For this review, take the finished solid that the model builds, in its own axes (mm). A direction names the side the tool comes from. Coordinates: 2 decimals unless noted, no trailing zeros. Order: outer loops, then holes, each group sorted by start corner. A loop starts at its lowest first (then second) coordinate and runs counter-clockwise, first axis right, second up. Notation, with made-up numbers: (2.25, 65) -> (34.25, 65) arc R34 ccw to (34.25, 101) -> close; hole circle Ø9 at (6.25, 47). An arc over 180 degrees is marked (long way). Answer as a JSON object with one key per item and string values. Group by question number.
1) Add section A-A, the plane z = 9.5. Write out the cut boundary in (x, y), then the cut area to 3 significant figures.
2) Wall thickness on L1, parallel to Y at x = 356.5, z = 1.95; L2, parallel to X at y = 387.5, z = 1.8; L3, parallel to X at y = 309, z = 9.5: over which ranges is each line inside the solid? List them lowest first.
3) Machinability: for faces 1 (the flat face through (173, 317, 3)), 2 (the flat face through (340, 388, 9)), 3 (the flat face through (179, 239.5, 6)), which of the approach directions +Z, -Z, +X, -X, +Y, -Y give a long, thin tool a straight path to every point of the face, cutting with its end or side? Answer none if there is none.
4) For pin 1 (3 mm diameter, centred on x = -5, y = 243.5, fed in from -Z); pin 2 (5 mm diameter, centred on x = 31.5, y = 335.5, fed in from +Z); pin 3 (10.5 mm diameter, centred on x = 328.5, y = 387, fed in from +Z), all flat-tipped, find the tip position at first contact; note any pin that passes through.
5) Add section C-C, the plane x = 237.5. Write out the cut boundary in (y, z), then the cut area to 3 significant figures.
6) Draft analysis for pull direction Y (two halves, no side actions). For faces 4 (the flat face through (173, 392.5, 6)), 5 (the flat face through (0, 317, 8)), 6 (the flat face through (-9.5, 315, 6)), state which applies: +Y half, -Y half, draft (parallel to the pull), parting line (faces both ways), or undercut.
7) Add section B-B, the plane y = 360. Write out the cut boundary in (x, z), then the cut area to 3 significant figures.
Autodesk Fusion 360 part; units mm, degrees
sketch "Sketch1" plane through (0, 0, 0) normal (0, 0, 1) x (1, 0, 0)
  line L0 (0, 250) -> (351, 250)
  line L1 (351, 250) -> (351, 383)
  line L2 (351, 383) -> (0, 383)
  line L3 (0, 383) -> (0, 250)
  line L4 (-9.5, 392.5) -> (361.5, 392.5)
  line L5 (361.5, 392.5) -> (361.5, 239.5)
  line L6 (361.5, 239.5) -> (-9.5, 239.5)
  line L7 (-9.5, 239.5) -> (-9.5, 392.5)
  circle A0 centre (-4.5, 244.5) radius 1.7
  circle A1 centre (356.5, 244.5) radius 1.7
  circle A2 centre (-4.5, 387.5) radius 1.7
  circle A3 centre (356.5, 387.5) radius 1.7
  circle A4 centre (-4.5, 387.5) radius 3
  circle A5 centre (356.5, 244.5) radius 3
  circle A6 centre (-4.5, 244.5) radius 3
  circle A7 centre (356.5, 387.5) radius 3
  dimension "d1" = 351
  dimension "d2" = 133
  dimension "d3" = 371
  dimension "d4" = 153
  dimension "d5" = 9.5
  dimension "d10" = 9.5
  dimension "d11" = 3.4
  dimension "d12" = 5
  dimension "d13" = 5
  dimension "d14" = 3.4
  dimension "d15" = 5
  dimension "d16" = 5
  dimension "d17" = 3.4
  dimension "d18" = 5
  dimension "d19" = 5
  dimension "d21" = 5
  dimension "d22" = 5
  dimension "d23" = 6
  dimension "d24" = 6
  dimension "d25" = 6
  dimension "d26" = 6
extrude "Extrude1" add sketch "Sketch1" along normal blind 10 from surface at 3.1 contours A4 | A5 | A6 | A7 makes body 1 at (-1.5928, 245.2403, 9.7667) makes body 2 at (357.3125, 247.3879, 9.7667) makes body 3 at (-7.0599, 389.0643, 9.7667) makes body 4 at (355.1314, 384.8304, 6.4333)
extrude "Extrude2" add sketch "Sketch1" along normal blind 13 contours L4 L5 L6 L7 bodies 1 2 3 4
extrude "Extrude3" add sketch "Sketch1" along normal blind 3 contours L0 L1 L2 L3 bodies 1
sketch "Sketch2" plane through (0, 0, 13) normal (0, 0, 1) x (-1, 0, 0)
  line L0 (0, -250) -> (0, -383)
  line L1 (0, -383) -> (-351, -383)
  line L2 (-351, -383) -> (-351, -250)
  line L3 (-351, -250) -> (0, -250)
  circle A0 centre (-356.5, -244.5) radius 3
  circle A1 centre (4.5, -244.5) radius 3
  circle A2 centre (4.5, -387.5) radius 3
  circle A3 centre (-356.5, -387.5) radius 3
  line L4 (9.5, -239.5) -> (-361.5, -239.5)
  line L5 (-361.5, -239.5) -> (-361.5, -392.5)
  line L6 (-361.5, -392.5) -> (9.5, -392.5)
  line L7 (9.5, -392.5) -> (9.5, -239.5)
sketch "Sketch3" plane through (0, 0, 13) normal (0, 0, 1) x (-1, 0, 0)
  line L0 (2440, -1230) -> (2470, -1230)
  line L1 (2470, -1230) -> (2470, -1260)
  line L2 (2470, -1260) -> (2440, -1260)
  line L3 (2440, -1260) -> (2440, -1230)
sketch "Sketch4" plane through (0, 0, 0) normal (1, 0, 0) x (0, 1, 0)
sketch "Sketch5" plane through (0, 0, 0) normal (0, 0, 1) x (1, 0, 0)
extrude "Extrude4" cut sketch "Sketch3" against normal blind 7.5 bodies 1
sketch "Sketch6" plane through (0, 0, 13) normal (0, 0, 1) x (-1, 0, 0)
  line L0 (-320, -400) -> (-340, -400)
  line L1 (-340, -400) -> (-340, -380)
  line L2 (-340, -380) -> (-320, -380)
  line L3 (-320, -380) -> (-320, -400)
extrude "Extrude5" cut sketch "Sketch6" against normal blind 7.5 bodies 1
Output values:
{
 "1": {"outline": "(-9.5, 239.5) -> (361.5, 239.5) -> (361.5, 392.5) -> (340, 392.5) -> (340, 383) -> (351, 383) -> (351, 250) -> (0, 250) -> (0, 383) -> (320, 383) -> (320, 392.5) -> (-9.5, 392.5) -> close; hole circle Ø3.4 at (-4.5, 244.5); hole circle Ø3.4 at (-4.5, 387.5); hole circle Ø3.4 at (356.5, 244.5); hole circle Ø3.4 at (356.5, 387.5)", "area": "9,850 mm²"},
 "2": {"L1": "y = 239.5 to 241.5, 247.5 to 384.5, 390.5 to 392.5", "L2": "x = -9.5 to -7.5, -1.5 to 353.5, 359.5 to 361.5", "L3": "x = -9.5 to 0, 351 to 361.5"},
 "3": {"face 1": "+Z", "face 2": "+Z, +Y", "face 3": "+Z, -Z, +X, -X, -Y"},
 "4": {"pin 1": "stops at z = 3.1", "pin 2": "stops at z = 3", "pin 3": "stops at z = 5.5"},
 "5": {"outline": "(239.5, 0) -> (392.5, 0) -> (392.5, 13) -> (383, 13) -> (383, 3) -> (250, 3) -> (250, 13) -> (239.5, 13) -> close", "area": "659 mm²"},
 "6": {"face 4": "+Y half", "face 5": "undercut", "face 6": "draft"},
 "7": {"outline": "(-9.5, 0) -> (361.5, 0) -> (361.5, 13) -> (351, 13) -> (351, 3) -> (0, 3) -> (0, 13) -> (-9.5, 13) -> close", "area": "1,310 mm²"}
}
